Study the drawing (mm; zero at the part's minimum x, y, z) and answer. A direction names the side the tool comes from. Round coordinates to 2 decimals unless told otherwise and drop trailing zeros. Order: outer loops, then holes, each group sorted by start corner. A loop starts at its lowest first (then second) coordinate and runs counter-clockwise, first axis right, second up. Notation, with made-up numbers: M 57,44 L 89,44 A26 ccw 89,69 Z; hole C 26,41.5 d5. An arc over 180 degrees is marked long. Put each result on its own line as item: value. Start each with the question number.
1. The mould has two halves that part along Z. Classify the marked faces 3, 4 and 5: +Z half, -Z half, draft (parallel to the pull), parting line (faces both ways), or undercut.
2. The part is cut by section C-C (x = 8.75). Give the vertices of the cut face in (y, z).
3. Which of the six approach directions +Z, -Z, +X, -X, +Y, -Y give full straight-line access (tool end or side, diameter ignored) to the marked faces 1 and 2?
4. Consider line 1 (Z direction, x = 4, y = 37.3); line 2 (X direction, y = 37, z = 15.5); line 3 (Z direction, x = 13.75, y = 24). Determine where each line is inside the solid, lowest interval first.
5. Each of these flat-tipped pins is pushed along its axis until it touches: pin 1 Ø6.5 at (x, z) = (4, 4) entering from -Y; pin 2 Ø10 at (x, y) = (14, 29) entering from -Z. Where does it stop, or does it pass through?
6. The part is cut by section D-D (y = 28.5). Give the vertices of the cut face in (x, z), then the cut area to 3 significant figures.
7. The part is cut by section B-B (z = 4). Give the vertices of the cut face in (x, y).
8. The part is cut by section A-A (x = 16). Give the vertices of the cut face in (y, z).
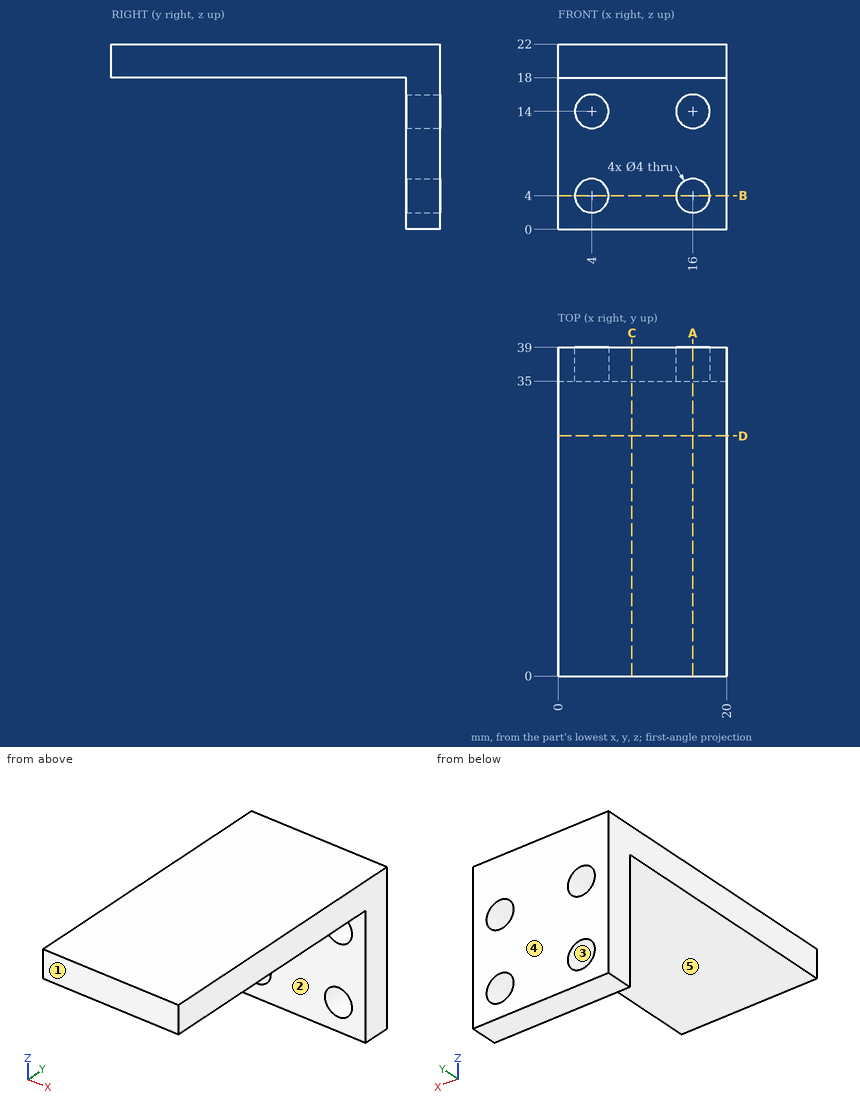
Resolved:
1. face 3: undercut
1. face 4: draft
1. face 5: -Z half
2. outline: M 0,18 L 35,18 L 35,0 L 39,0 L 39,22 L 0,22 Z
3. face 1: +Z, -Z, +X, -X, -Y
3. face 2: -Z, +X, -X, -Y
4. line 1: 0 to 2, 6 to 12, 16 to 22
4. line 2: 0 to 2.68, 5.32 to 14.68, 17.32 to 20
4. line 3: 18 to 22
5. pin 1: y = 35
5. pin 2: z = 18
6. outline: M 0,18 L 20,18 L 20,22 L 0,22 Z
6. area: 80.0 mm2
7. outline: M 0,35 L 2,35 L 2,39 L 0,39 Z; M 6,35 L 14,35 L 14,39 L 6,39 Z; M 18,35 L 20,35 L 20,39 L 18,39 Z
8. outline: M 0,18 L 35,18 L 35,16 L 39,16 L 39,22 L 0,22 Z; M 35,0 L 39,0 L 39,2 L 35,2 Z; M 35,6 L 39,6 L 39,12 L 35,12 Z
